```python
from build123d import *

# Parameters (mm, degrees)
ESBO_O1_W                                            = 42
ESBO_O1_H                                            = 65
RESSALTO_EXTRUS_O1_DEPTH                             = 21
ESBO_O2_W                                            = 17
ESBO_O2_H                                            = 22.225
CORTE_EXTRUS_O1_DEPTH                                = 43
FURO_COM_FOLGA_DE_M31_D                              = 3.4544
FURO_COM_FOLGA_DE_M31_DEPTH                          = 21
FURO_COM_FOLGA_DE_M201_D                             = 22.225
FURO_COM_FOLGA_DE_M201_DEPTH                         = 21
REBAIXO_PARA_PARAFUSO_DE_M_QUINA_DE_CABE_D           = 3.2
REBAIXO_PARA_PARAFUSO_DE_M_QUINA_DE_CABE_DEPTH       = 21
REBAIXO_PARA_PARAFUSO_DE_M_QUINA_DE_CABE_CBORE_D     = 6
REBAIXO_PARA_PARAFUSO_DE_M_QUINA_DE_CABE_CBORE_DEPTH = 7.62
FURO1_D                                              = 8.334375
FURO1_DEPTH                                          = 8
ESBO_O11_W                                           = 42
ESBO_O11_H                                           = 65
ESBO_O11_R                                           = 11.1125
ESBO_O11_R_2                                         = 1.7272
ESBO_O11_R_3                                         = 1.6
RESSALTO_EXTRUS_O2_DEPTH                             = 4
ESBO_O13_R                                           = 11.1125
ESBO_O13_R_2                                         = 5
RESSALTO_EXTRUS_O3_DEPTH                             = 5


with BuildPart() as part:
    # Esboço1 → Ressalto-extrusão1 (new body)
    with BuildSketch(Plane.XY.offset(21)):
        with Locations((21, 32.5)):
            Rectangle(ESBO_O1_W, ESBO_O1_H)
    extrude(amount=-RESSALTO_EXTRUS_O1_DEPTH)

    # Esboço2 → Corte-extrusão1 (cut, through all)
    with BuildSketch(Plane(origin=(42, 0, 0), x_dir=(0, 0, -1), z_dir=(1, 0, 0))):
        with Locations((-8.5, 32.5)):
            Rectangle(ESBO_O2_W, ESBO_O2_H)
    extrude(amount=-CORTE_EXTRUS_O1_DEPTH, mode=Mode.SUBTRACT)

    # Furo com folga de M31
    with Locations(Plane(origin=(0, 0, 0), x_dir=(-1, 0, 0), z_dir=(0, 0, -1))):
        with Locations((-30, 7), (-16.7, 7), (-16.7, 58), (-30, 58)):
            Hole(FURO_COM_FOLGA_DE_M31_D / 2, depth=FURO_COM_FOLGA_DE_M31_DEPTH)

    # Furo com folga de M201
    with Locations(Plane.XY.offset(21)):
        with Locations((21, 32.5)):
            Hole(FURO_COM_FOLGA_DE_M201_D / 2, depth=FURO_COM_FOLGA_DE_M201_DEPTH)

    # Rebaixo para parafuso de máquina de cabeça sextavada de M31
    with Locations(Plane(origin=(0, 0, 0), x_dir=(-1, 0, 0), z_dir=(0, 0, -1))):
        with Locations((-36.5, 17), (-5.5, 17), (-5.5, 48), (-36.5, 48)):
            CounterBoreHole(REBAIXO_PARA_PARAFUSO_DE_M_QUINA_DE_CABE_D / 2, REBAIXO_PARA_PARAFUSO_DE_M_QUINA_DE_CABE_CBORE_D / 2, REBAIXO_PARA_PARAFUSO_DE_M_QUINA_DE_CABE_CBORE_DEPTH, depth=REBAIXO_PARA_PARAFUSO_DE_M_QUINA_DE_CABE_DEPTH)

    # Furo1
    with Locations(Plane(origin=(42, 0, 0), x_dir=(0, 0, -1), z_dir=(1, 0, 0))):
        with Locations((-14, 7), (-14, 58)):
            Hole(FURO1_D / 2, depth=FURO1_DEPTH)

    # Esboço11 → Ressalto-extrusão2 (add)
    with BuildSketch(Plane.XY.offset(21)):
        with Locations((21, 32.5)):
            Rectangle(ESBO_O11_W, ESBO_O11_H)
        with Locations((21, 32.5)):
            Circle(ESBO_O11_R, mode=Mode.SUBTRACT)
        with Locations((16.7, 7)):
            Circle(ESBO_O11_R_2, mode=Mode.SUBTRACT)
        with Locations((30, 7)):
            Circle(ESBO_O11_R_2, mode=Mode.SUBTRACT)
        with Locations((5.5, 17)):
            Circle(ESBO_O11_R_3, mode=Mode.SUBTRACT)
        with Locations((5.5, 48)):
            Circle(ESBO_O11_R_3, mode=Mode.SUBTRACT)
        with Locations((16.7, 58)):
            Circle(ESBO_O11_R_2, mode=Mode.SUBTRACT)
        with Locations((36.5, 48)):
            Circle(ESBO_O11_R_3, mode=Mode.SUBTRACT)
        with Locations((30, 58)):
            Circle(ESBO_O11_R_2, mode=Mode.SUBTRACT)
        with Locations((36.5, 17)):
            Circle(ESBO_O11_R_3, mode=Mode.SUBTRACT)
    extrude(amount=RESSALTO_EXTRUS_O2_DEPTH)

    # Esboço13 → Ressalto-extrusão3 (add)
    with BuildSketch(Plane(origin=(0, 0, 17), x_dir=(-1, 0, 0), z_dir=(0, 0, -1))):
        with Locations((-21, 32.5)):
            Circle(ESBO_O13_R)
        with Locations((-21, 32.5)):
            Circle(ESBO_O13_R_2, mode=Mode.SUBTRACT)
    extrude(amount=-RESSALTO_EXTRUS_O3_DEPTH)


solid = part.part
```
Can you work these out from the model? Positions are in its coordinate system, mm. A direction names the side the tool comes from. Round coordinates to 2 decimals unless told otherwise and drop trailing zeros. Loops run counter-clockwise (first coordinate to the right, second up) from the corner with the lowest first, then second, coordinate; pieces in that order, holes last. Notation, with made-up numbers: M 39.25,-23.5 L 86.25,-23.5 A8 cw 86.25,-9.5 Z; hole C 61.25,-22.5 d6. An arc over 180 degrees is marked long. Answer as a JSON object with one key per item and string values. Group by question number.
Q1. Please list where these lines run through material, in increasing order: L1, parallel to Y at x = 36.5, z = 4.25; L2, parallel to Y at x = 5.5, z = 22.8; L3, parallel to Y at x = 30, z = 9.5.
Q2. Imagine slicing it at C-C, the plane y = 32.5. Please give me the cut outline in (x, z), then the cut area to 3 significant figures.
Q3. We'd pull the mould along Y, two halves only. Please class faces 1 (the cylindrical face through (37.944, 8.252, 17.975)), 2 (the flat face through (30, 25.7, 25)): +Y half, -Y half, draft (parallel to the pull), parting line (faces both ways), or undercut.
Q4. Imagine slicing it at B-B, the plane x = 36.5. Please give me the cut outline in (y, z).
Q5. Imagine slicing it at A-A, the plane z = 4.5. Count the separate pieces of the cut face and the enclosed holes in it, then the cut area to 3 significant figures.
Q6. Will these pins go through, and if not, where does the flat tip stop? pin 1 (5 mm diameter, centred on x = 36.5, y = 17, fed in from +Z); pin 2 (5 mm diameter, centred on x = 5.5, y = 17, fed in from -Z); pin 3 (3 mm diameter, centred on x = 30, y = 7, fed in from +Z).
Q7. On a 3-axis mill with a long thin cutter (end or side, diameter ignored), from which of +Z, -Z, +X, -X, +Y, -Y can I reach the whole of each face in a straight line? I mean faces 3 (the flat face through (42, 32, 18)), 4 (the cylindrical face through (6.15, 14.07, 3.76)), 5 (the flat face through (18.7, 27.7, 22)), 6 (the flat face through (21, 43.612, 9)), 7 (the flat face through (34, 7, 14)). Say none if no direction works.
Findings:
{
 "1": {"L1": "y = 0 to 14, 20 to 21.39, 43.61 to 45, 51 to 65", "L2": "y = 0 to 15.4, 18.6 to 46.4, 49.6 to 65", "L3": "y = 0 to 5.27, 8.73 to 21.39, 43.61 to 56.27, 59.73 to 65"},
 "2": {"outline": "M 0,17 L 16,17 L 16,22 L 9.89,22 L 9.89,25 L 0,25 Z; M 26,17 L 42,17 L 42,25 L 32.11,25 L 32.11,22 L 26,22 Z", "area": "219 mm2"},
 "3": {"face 1": "undercut", "face 2": "draft"},
 "4": {"outline": "M 0,0 L 14,0 L 14,7.62 L 15.4,7.62 L 15.4,25 L 0,25 Z; M 18.6,7.62 L 20,7.62 L 20,0 L 21.39,0 L 21.39,17 L 43.61,17 L 43.61,0 L 45,0 L 45,7.62 L 46.4,7.62 L 46.4,25 L 18.6,25 Z; M 49.6,7.62 L 51,7.62 L 51,0 L 65,0 L 65,25 L 49.6,25 Z; hole C 7,14 d8.33; hole C 58,14 d8.33"},
 "5": {"separate pieces": "2", "enclosed holes": "8", "area": "1,650 mm2"},
 "6": {"pin 1": "stops at z = 25", "pin 2": "stops at z = 7.62", "pin 3": "passes through"},
 "7": {"face 3": "+Z, -Z, +X, +Y, -Y", "face 4": "-Z", "face 5": "+Z", "face 6": "-Z, +X, -X", "face 7": "+X"}
}
